Could you check a few things on this model? Use its own coordinates, in mm. Round coordinates to 2 decimals unless told otherwise and drop trailing zeros. Loops run counter-clockwise (first coordinate to the right, second up) from the corner with the lowest first, then second, coordinate; pieces in that order, holes last. Notation, with made-up numbers: (47, 18.5) -> (74, 18.5) arc R29 ccw to (74, 42.5) -> close; hole circle Ø6 at (-3.5, 82.25). An arc over 180 degrees is marked (long way). One line per item, written item: value.
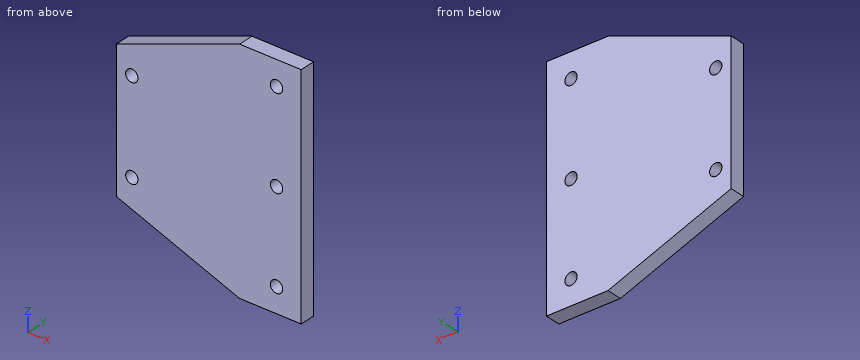
```python
from build123d import *

# Parameters (mm, degrees)
BOSS_EXTRUDE1_OUTLINE_W = 120
BOSS_EXTRUDE1_OUTLINE_H = 150
BOSS_EXTRUDE1_DEPTH     = 10
CHAMFER1_SIZE           = 30
CHAMFER1_SIZE2          = 80
CHAMFER2_SIZE           = 80
CHAMFER2_SIZE2          = 30
SKETCH2_R               = 4
CUT_EXTRUDE1_DEPTH      = 10
SCALE1_SCALE            = 7.5


# Read off the part's stored shape, not the designer's step: Boss-Extrude1
with BuildPart() as part:
    # Boss-Extrude1 outline → Boss-Extrude1 (new body)
    with BuildSketch(Plane(origin=(0, 0, 0), x_dir=(1, 0, 0), z_dir=(0, 1, 0))):
        with Locations((60, 75)):
            Rectangle(BOSS_EXTRUDE1_OUTLINE_W, BOSS_EXTRUDE1_OUTLINE_H)
    extrude(amount=BOSS_EXTRUDE1_DEPTH)

    # Chamfer1
    chamfer1_edges = [part.edges().sort_by_distance(p)[0] for p in [
        (0, 5, 0),
    ]]
    chamfer1_side = [part.faces().sort_by_distance(p)[0] for p in [
        (0, 5, -75),
    ]]
    chamfer(chamfer1_edges, length=CHAMFER1_SIZE, length2=CHAMFER1_SIZE2, reference=chamfer1_side[0])

    # Chamfer2
    chamfer2_edges = [part.edges().sort_by_distance(p)[0] for p in [
        (0, 5, -150),
    ]]
    chamfer2_side = [part.faces().sort_by_distance(p)[0] for p in [
        (60, 5, -150),
    ]]
    chamfer(chamfer2_edges, length=CHAMFER2_SIZE, length2=CHAMFER2_SIZE2, reference=chamfer2_side[0])

    # Sketch2 → Cut-Extrude1 (cut)
    with BuildSketch(Plane(origin=(0, 10, 0), x_dir=(1, 0, 0), z_dir=(0, 1, 0))):
        with Locations(Location((104, 134, 0), (0, 0, 270))):
            Circle(SKETCH2_R)
        with Locations(Location((104, 16, 0), (0, 0, 270))):
            Circle(SKETCH2_R)
        with Locations(Location((10, 105, 0), (0, 0, 270))):
            Circle(SKETCH2_R)
        with Locations(Location((10, 45, 0), (0, 0, 270))):
            Circle(SKETCH2_R)
        with Locations(Location((104, 75, 0), (0, 0, 270))):
            Circle(SKETCH2_R)
    extrude(amount=-CUT_EXTRUDE1_DEPTH, mode=Mode.SUBTRACT)


with BuildPart() as part_1:
    # Scale1: scaled about (65.107380076, 5, -75)
    add(part.part.scale(SCALE1_SCALE).moved(Location((-423.197970494, -32.5, 487.5))))


solid = part_1.part
```
Item 1: I need wall thicknesses on line 1 (Z direction, x = -336.5, y = 17); line 2 (X direction, y = 1, z = 150); line 3 (X direction, y = -25.5, z = -68.5). Which ranges of each line are inside material? Lowest first, please. Write a range as from..to.
Output:
line 1: z = -445.01..-327.63, -272.37..122.37, 177.63..295.01
line 2: x = -423.2..-378.2, -318.2..476.8
line 3: x = -423.2..327.51, 386.09..476.8
Item 2: If we section it at C-C on z = 157.5: List the corners of the cut face in (x, y) for me, plus the area to 3 significant figures.
Output:
outline: (-423.2, -32.5) -> (-377.25, -32.5) -> (-377.25, 42.5) -> (-423.2, 42.5) -> close; (-319.15, -32.5) -> (476.8, -32.5) -> (476.8, 42.5) -> (-319.15, 42.5) -> close
area: 63,100 mm²
Item 3: Will these pins go through, and if not, where does the flat tip stop? pin 1 Ø10 at (x, y) = (-185.5, -8) entering from +Z; pin 2 Ø10 at (x, y) = (-294.5, -12) entering from +Z.
Output:
pin 1: stops at z = 353.51
pin 2: stops at z = 312.64
Item 4: If we section it at A-A on z = -75: List the corners of the cut face in (x, y) for me, plus the area to 3 significant figures.
Output:
outline: (-423.2, -32.5) -> (326.8, -32.5) -> (326.8, 42.5) -> (-423.2, 42.5) -> close; (386.8, -32.5) -> (476.8, -32.5) -> (476.8, 42.5) -> (386.8, 42.5) -> close
area: 63,000 mm²
Item 5: If we section it at D-D on x = 54: List the corners of the cut face in (y, z) for me, plus the area to 3 significant figures.
Output:
outline: (-32.5, -591.45) -> (42.5, -591.45) -> (42.5, 441.45) -> (-32.5, 441.45) -> close
area: 77,500 mm²
Item 6: If we section it at B-B on y = 31: List the corners of the cut face in (x, z) for me, plus the area to 3 significant figures.
Output:
outline: (-423.2, -412.5) -> (176.8, -637.5) -> (476.8, -637.5) -> (476.8, 487.5) -> (176.8, 487.5) -> (-423.2, 262.5) -> close; hole circle Ø60 at (-348.2, -300); hole circle Ø60 at (-348.2, 150); hole circle Ø60 at (356.8, -517.5); hole circle Ø60 at (356.8, -75); hole circle Ø60 at (356.8, 367.5)
area: 863,000 mm²
